```python
from build123d import *

# Parameters (mm, degrees)
BOSS_EXTRUDE1_DEPTH          = 1.5875
SKETCH7_W                    = 1.5875
SKETCH7_H                    = 101.6
BOSS_EXTRUDE2_DEPTH          = 0.0254
EDGE_FLANGE1_STRIP_W         = 19.05
EDGE_FLANGE1_STRIP_H         = 1.5875
EDGE_FLANGE1_STRIP_CUT_DEPTH = 101.6
EDGE_FLANGE1_DEPTH           = 101.6
SKETCH11_W                   = 101.6
SKETCH11_H                   = 1.5875
BOSS_EXTRUDE3_DEPTH          = 0.0254
EDGE_FLANGE2_STRIP_W         = 19.05
EDGE_FLANGE2_STRIP_H         = 1.5875
EDGE_FLANGE2_STRIP_CUT_DEPTH = 101.6
EDGE_FLANGE2_DEPTH           = 101.6
SKETCH15_R                   = 3.175
CUT_EXTRUDE1_DEPTH           = 2.54
SKETCH16_R                   = 3.175
CUT_EXTRUDE2_DEPTH           = 2.54


# Sheet-metal steps are written as plain solids
with BuildPart() as part:
    # Sketch1 → Boss-Extrude1 (new body)
    with BuildSketch(Plane.XY):
        Polygon((0, 119.481843199), (0, -32.918156801), (152.4, -32.918156801), align=None)
    extrude(amount=BOSS_EXTRUDE1_DEPTH)

    # Sketch7 → Boss-Extrude2 (add)
    with BuildSketch(Plane.ZY):
        with Locations((0.79375, 43.281843199)):
            Rectangle(SKETCH7_W, SKETCH7_H)
    extrude(amount=BOSS_EXTRUDE2_DEPTH)

    # Edge-Flange1 strip (across the edge) → Edge-Flange1 strip cut (cut)
    with BuildSketch(Plane(origin=(-0.0254, 94.081843199, 1.5875), x_dir=(1, 0, 0), z_dir=(0, -1, 0))):
        with Locations((-1.5875, -0.79375)):
            Rectangle(EDGE_FLANGE1_STRIP_W, EDGE_FLANGE1_STRIP_H)
    extrude(amount=EDGE_FLANGE1_STRIP_CUT_DEPTH, mode=Mode.SUBTRACT)

    # Edge-Flange1 section (across the edge) → Edge-Flange1 (add)
    with BuildSketch(Plane(origin=(-0.0254, 94.081843199, 1.5875), x_dir=(1, 0, 0), z_dir=(0, -1, 0))):
        with BuildLine():
            Line((0, 6.35), (0, 23.8125))
            Line((0, 23.8125), (1.5875, 23.8125))
            Line((1.5875, 23.8125), (1.5875, 6.35))
            ThreePointArc((1.5875, 6.35), (3.447371939, 1.859871939), (7.9375, 0))
            Line((7.9375, 0), (7.9375, -1.5875))
            ThreePointArc((7.9375, -1.5875), (2.324839924, 0.737339924), (0, 6.35))
        make_face()
    extrude(amount=EDGE_FLANGE1_DEPTH)

    # Sketch11 → Boss-Extrude3 (add)
    with BuildSketch(Plane(origin=(0, -32.918156801, 0), x_dir=(-1, 0, 0), z_dir=(0, -1, 0))):
        with Locations((-76.2, -0.79375)):
            Rectangle(SKETCH11_W, SKETCH11_H)
    extrude(amount=BOSS_EXTRUDE3_DEPTH)

    # Edge-Flange2 strip (across the edge) → Edge-Flange2 strip cut (cut)
    with BuildSketch(Plane(origin=(25.4, -32.943556801, 1.5875), x_dir=(0, 1, 0), z_dir=(1, 0, 0))):
        with Locations((-1.5875, -0.79375)):
            Rectangle(EDGE_FLANGE2_STRIP_W, EDGE_FLANGE2_STRIP_H)
    extrude(amount=EDGE_FLANGE2_STRIP_CUT_DEPTH, mode=Mode.SUBTRACT)

    # Edge-Flange2 section (across the edge) → Edge-Flange2 (add)
    with BuildSketch(Plane(origin=(25.4, -32.943556801, 1.5875), x_dir=(0, 1, 0), z_dir=(1, 0, 0))):
        with BuildLine():
            Line((0, 6.35), (0, 23.8125))
            Line((0, 23.8125), (1.5875, 23.8125))
            Line((1.5875, 23.8125), (1.5875, 6.35))
            ThreePointArc((1.5875, 6.35), (3.447371939, 1.859871939), (7.9375, 0))
            Line((7.9375, 0), (7.9375, -1.5875))
            ThreePointArc((7.9375, -1.5875), (2.324839924, 0.737339924), (0, 6.35))
        make_face()
    extrude(amount=EDGE_FLANGE2_DEPTH)

    # Sketch15 → Cut-Extrude1 (cut)
    with BuildSketch(Plane(origin=(0, -31.356056801, 0), x_dir=(1, 0, 0), z_dir=(0, 1, 0))):
        with Locations(Location((38.1, -19.05, 0), (0, 0, 270))):
            Circle(SKETCH15_R)
        with Locations(Location((63.5, -19.05, 0), (0, 0, 270))):
            Circle(SKETCH15_R)
        with Locations(Location((88.9, -19.05, 0), (0, 0, 270))):
            Circle(SKETCH15_R)
        with Locations(Location((114.3, -19.05, 0), (0, 0, 270))):
            Circle(SKETCH15_R)
    extrude(amount=-CUT_EXTRUDE1_DEPTH, mode=Mode.SUBTRACT)

    # Sketch16 → Cut-Extrude2 (cut)
    with BuildSketch(Plane(origin=(1.5621, 0, 0), x_dir=(0, 0, -1), z_dir=(1, 0, 0))):
        with Locations((-19.05, 81.381843199)):
            Circle(SKETCH16_R)
        with Locations((-19.05, 55.981843199)):
            Circle(SKETCH16_R)
        with Locations((-19.05, 30.581843199)):
            Circle(SKETCH16_R)
        with Locations((-19.05, 5.181843199)):
            Circle(SKETCH16_R)
    extrude(amount=-CUT_EXTRUDE2_DEPTH, mode=Mode.SUBTRACT)


solid = part.part
```
Model file for the job. Use its own axes, mm. A direction names the side the tool comes from. Coordinates: 2 decimals unless noted, no trailing zeros. Loops run counter-clockwise (first coordinate to the right, second up) from the corner with the lowest first, then second, coordinate; pieces in that order, holes last. Notation, with made-up numbers: (78.5, 89) -> (86.5, 89) arc R32 cw to (86.5, 119) -> close; hole circle Ø7 at (79, -27). An arc over 180 degrees is marked (long way). Answer as a JSON object with one key per item and string values.
Q1. Cut at A-A (z = 12). List the corners of the cut face in (x, y), and give its area (3 significant figures).
Report:
{"outline": "(-0.03, -7.52) -> (1.56, -7.52) -> (1.56, 94.08) -> (-0.03, 94.08) -> close; (25.4, -32.94) -> (127, -32.94) -> (127, -31.36) -> (25.4, -31.36) -> close", "area": "323 mm2"}
Q2. Pull direction X, two halves, no side cores. Call faces 6 (the flat face through (25.4, -32, 13)), 7 (the cylindrical face through (65.646, -32.139, 16.71)), 8 (the flat face through (77.267, 42.215, 0.783)): released by +X, released by -X, zero draft, split by the parting line, or undercut.
Report:
{"face 6": "released by -X", "face 7": "undercut", "face 8": "released by +X"}
Q3. Probe probe 1 along Y at (x, z) = (1, 19.05); probe 2 along X at (y, z) = (-32.1, 19.05) (3 decimals); probe 3 along Y at (x, z) = (110, 9.5). List the from-to ranges inside material, lowest first.
Report:
{"probe 1": "y = -7.52 to 2.01, 8.36 to 27.41, 33.76 to 52.81, 59.16 to 78.21, 84.56 to 94.08", "probe 2": "x = 25.4 to 34.925, 41.275 to 60.325, 66.675 to 85.725, 92.075 to 111.125, 117.475 to 127", "probe 3": "y = -32.94 to -31.36"}
Q4. 3-axis set-ups, long thin cutter, end or side, ignore diameter. For faces 1 (the cylindrical face through (2.361, 43.993, 2.263)), 2 (the flat face through (-0.025, 44, 17)), 3 (the flat face through (75, -31.356, 17)), 4 (the cylindrical face through (75.489, -30.557, 2.263)), 5 (the cylindrical face through (111.2, -32.14, 18.36)): which of +Z, -Z, +X, -X, +Y, -Y reach the whole face in a straight line?
Report:
{"face 1": "-Z, -X", "face 2": "+Z, -Z, -X, +Y, -Y", "face 3": "+Z, +X, -X, +Y", "face 4": "-Z, -Y", "face 5": "+Y, -Y"}
Q5. Flat gauge pins, fed straight in: P1, Ø1.7, axis at y = 109.5, z = 0.5, coming from the -X side; P2, Ø3, axis at x = 27, y = 7.5, coming from the +Z side; P3, Ø1.7, axis at x = 142, z = 1, coming from the -Y side; P4, Ø5.5, axis at y = 30.58, z = 19.05, coming from the +X side. Where does each tip first touch, or does it go through?
Report:
{"P1": "stops at x = 0", "P2": "stops at z = 1.59", "P3": "stops at y = -32.92", "P4": "passes through"}
